Model file for the job. Use its own axes, mm. A direction names the side the tool comes from. Coordinates: 2 decimals unless noted, no trailing zeros. Order: outer loops, then holes, each group sorted by start corner. A loop starts at its lowest first (then second) coordinate and runs counter-clockwise, first axis right, second up. Notation, with made-up numbers: (28.5, -17.5) -> (38.5, -17.5) arc R22 ccw to (38.5, -5.5) -> close; hole circle Ø1 at (-39, 0). An arc over 180 degrees is marked (long way). Use CSV: the item, a comma, the result in double quotes. Start each with the question number.
(1) Cut at C-C on y = 22. Write the cut outline in (x, z), plus the area to 3 significant figures.
(2) Pin check, flat tips, straight feed: pin 1 Ø2.5 at (y, z) = (5, 0) entering from -X; pin 2 Ø3 at (x, z) = (1, 0.5) entering from +Y. Stop position of each tip, or through.
(3) Cut at B-B on y = 5. Write the cut outline in (x, z), plus the area to 3 significant figures.
(4) Probe L1, parallel to Y at x = 4.5, z = 0; L2, parallel to Y at x = -1.5, z = 4.5; L3, parallel to Y at x = 2.5, z = -1. List the from-to ranges inside material, lowest first.
(5) Cut at A-A on y = 27. Write the cut outline in (x, z), plus the area to 3 significant figures.
(6) Tool access for faces 1 (the cylindrical face through (0, 28, 5)), 2 (the flat face through (0, 33, 3)): list every direction of +Z, -Z, +X, -X, +Y, -Y with a clear straight run to the whole face (end or side of a thin tool).
```python
from build123d import *

# Parameters (mm, degrees)
SKETCH1_R               = 6
BOSS_EXTRUDE1_DEPTH     = 23
SKETCH2_R               = 2
BOSS_EXTRUDE2_DEPTH     = 10
SKETCH3_R               = 1.5
CUT_EXTRUDE1_DEPTH      = 7
CUT_EXTRUDE1_DEPTH_BACK = 7
CHAMFER1_SIZE           = 0.25
CHAMFER1_SIZE2          = 0.433012702
CHAMFER2_SIZE           = 0.5
CHAMFER2_SIZE2          = 0.866025404
CHAMFER2_PART_2_SIZE    = 0.5
CHAMFER2_PART_2_SIZE2   = 0.866025404


with BuildPart() as part:
    # Sketch1 → Boss-Extrude1 (new body)
    with BuildSketch(Plane(origin=(0, 0, 0), x_dir=(1, 0, 0), z_dir=(0, 1, 0))):
        Circle(SKETCH1_R)
    extrude(amount=BOSS_EXTRUDE1_DEPTH)

    # Sketch2 → Boss-Extrude2 (add)
    with BuildSketch(Plane(origin=(0, 23, 0), x_dir=(1, 0, 0), z_dir=(0, 1, 0))):
        with Locations((0, -3)):
            Circle(SKETCH2_R)
    extrude(amount=BOSS_EXTRUDE2_DEPTH)

    # Sketch3 → Cut-Extrude1 (cut, two sides)
    with BuildSketch(Plane(origin=(0, 0, 0), x_dir=(0, 0, -1), z_dir=(1, 0, 0))) as cut_extrude1_sk:
        with Locations((0, 5)):
            Circle(SKETCH3_R)
    extrude(amount=CUT_EXTRUDE1_DEPTH, mode=Mode.SUBTRACT)
    extrude(cut_extrude1_sk.sketch, amount=-CUT_EXTRUDE1_DEPTH_BACK, mode=Mode.SUBTRACT)

    # Chamfer1
    chamfer1_edges = [part.edges().sort_by_distance(p)[0] for p in [
        (-2, 33, 3),
    ]]
    chamfer1_side = [part.faces().sort_by_distance(p)[0] for p in [
        (-2, 28, 3),
    ]]
    chamfer(chamfer1_edges, length=CHAMFER1_SIZE, length2=CHAMFER1_SIZE2, reference=chamfer1_side[0])

    # Chamfer2
    chamfer2_edges = [part.edges().sort_by_distance(p)[0] for p in [
        (-6, 0, 0),
    ]]
    chamfer2_side = [part.faces().sort_by_distance(p)[0] for p in [
        (0, 0, 0),
    ]]
    chamfer(chamfer2_edges, length=CHAMFER2_SIZE, length2=CHAMFER2_SIZE2, reference=chamfer2_side[0])

    # Chamfer2 part 2
    chamfer2_part_2_edges = [part.edges().sort_by_distance(p)[0] for p in [
        (-6, 23, 0),
    ]]
    chamfer2_part_2_side = [part.faces().sort_by_distance(p)[0] for p in [
        (-6, 11.5, 0),
    ]]
    chamfer(chamfer2_part_2_edges, length=CHAMFER2_PART_2_SIZE, length2=CHAMFER2_PART_2_SIZE2, reference=chamfer2_part_2_side[0])


solid = part.part
```
Outcome:
1,outline,"circle Ø12 at (0, 0)"
1,area,"113 mm2"
2,pin 1,"through"
2,pin 2,"y = 33"
3,outline,"(-5.81, -1.5) arc R6 ccw to (5.81, -1.5) -> close; (-5.81, 1.5) -> (5.81, 1.5) arc R6 ccw to start"
3,area,"77.5 mm2"
4,L1,"0 to 3.5, 6.5 to 23"
4,L2,"0 to 23"
4,L3,"0 to 3.88, 6.12 to 23"
5,outline,"circle Ø4 at (0, 3)"
5,area,"12.6 mm2"
6,face 1,"+Y"
6,face 2,"+Z, -Z, +X, -X, +Y"
